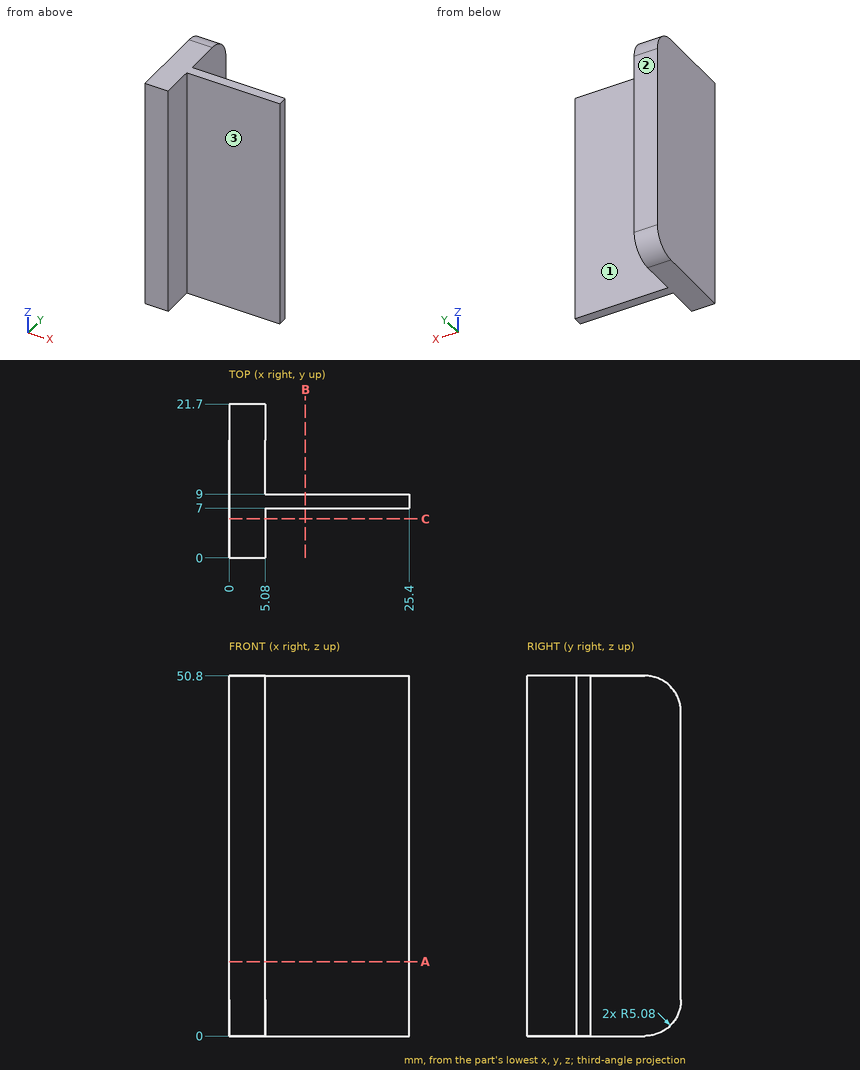
Geometry check sheet. Reference: drawing and pictorial views, mm from the part's lowest x, y, z. A direction names the side the tool comes from. Round coordinates to 2 decimals unless told otherwise and drop trailing zeros. Loops run counter-clockwise (first coordinate to the right, second up) from the corner with the lowest first, then second, coordinate; pieces in that order, holes last. Notation, with made-up numbers: (40.5, 61) - (97.5, 61) arc R24 ccw to (97.5, 81) - close; hole circle Ø3 at (31, 9). An arc over 180 degrees is marked (long way). Answer in a Markdown table with one row per item. Add a question column.
Q1. Section check A-A on z = 10.5. Enter the section's corners in (x, y), plus the area to 3 significant figures.
Q2. Section check C-C on y = 5.5. Enter the section's corners in (x, z), plus the area to 3 significant figures.
Q3. Tool access check on the marked faces 1, 2 and 3. Record the directions out of +Z, -Z, +X, -X, +Y, -Y that give a thin tool (end or side, any length) a straight path to the whole face; none if there is none.
Q4. Gauge pin test, flat ends, axial feed: pin 1 (3 mm diameter, centred on y = 2.5, z = 44.5, fed in from +X); pin 2 (8 mm diameter, centred on x = 12.5, z = 27.5, fed in from -Y); pin 3 (1.5 mm diameter, centred on x = 16.5, z = 20.5, fed in from +Y). Record the tip position at first contact, or that the pin passes through.
Q5. Section check B-B on x = 10.75. Enter the section's corners in (y, z), plus the area to 3 significant figures.
Q6. Material ranges on line 1 (X direction, y = 6.5, z = 35); line 2 (Y direction, x = 21.25, z = 31); line 3 (Z direction, x = 2.5, y = 20.25), recorded low to high.
Found:
| question | item | result |
|---|---|---|
| 1 | outline | (0, 0) - (5.08, 0) - (5.08, 7) - (25.4, 7) - (25.4, 9) - (5.08, 9) - (5.08, 21.7) - (0, 21.7) - close |
| 1 | area | 151 mm² |
| 2 | outline | (0, 0) - (5.08, 0) - (5.08, 50.8) - (0, 50.8) - close |
| 2 | area | 258 mm² |
| 3 | face 1 | +Z, -Z, +X, +Y |
| 3 | face 2 | +Z, -Z, +X, -X, +Y |
| 3 | face 3 | +Z, -Z, +X, -Y |
| 4 | pin 1 | stops at x = 5.08 |
| 4 | pin 2 | stops at y = 7 |
| 4 | pin 3 | stops at y = 9 |
| 5 | outline | (7, 0) - (9, 0) - (9, 50.8) - (7, 50.8) - close |
| 5 | area | 102 mm² |
| 6 | line 1 | x = 0 to 5.08 |
| 6 | line 2 | y = 7 to 9 |
| 6 | line 3 | z = 1.53 to 49.27 |
